Could you check a few things on this drawing? It's one solid part, dimensions in mm from its lowest x, y, z. A direction names the side the tool comes from. Give positions to 0.01 mm unless a question says otherwise; leave off trailing zeros. Order: outer loops, then holes, each group sorted by start corner. A loop starts at its lowest first (then second) coordinate and runs counter-clockwise, first axis right, second up.
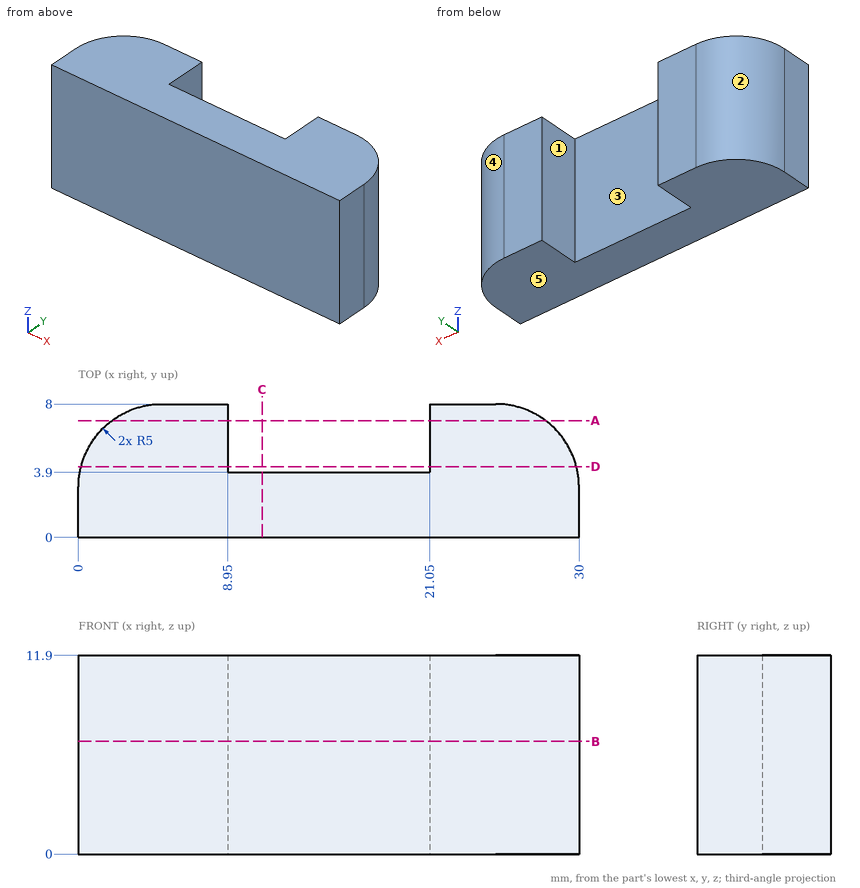
1) Suppose I cut it at C-C (x = 11). Please give me the cut outline in (y, z), and give its area (3 significant figures).
2) Suppose I cut it at A-A (y = 7). Please give me the cut outline in (x, z), and give its area (3 significant figures).
3) Suppose I cut it at D-D (y = 4.25). Please give me the cut outline in (x, z), and give its area (3 significant figures).
4) Which directions (+Z, -Z, +X, -X, +Y, -Y) give clear straight access to the entire face, cutting with the end or side of a thin tool? Please do the marked faces 1 and 2.
5) If I drill on line 1 (Y direction, x = 9.25, z = 5.5); line 2 (X direction, y = 6, z = 1.5); line 3 (X direction, y = 7, z = 11.25), over which ranges is the centre line in solid material (lowest first)?
6) I'm going to push flat-ended pins straight in: pin 1 Ø3.5 at (y, z) = (6, 5) entering from +X; pin 2 Ø4.5 at (y, z) = (5.5, 3) entering from -X; pin 3 Ø3.5 at (x, z) = (16, 6) entering from +Y. Where does each tip first touch, or does it pass through?
7) We'd pull the mould along X, two halves only. Please class the marked faces 3, 4 and 5: +X half, -X half, draft (parallel to the pull), parting line (faces both ways), or undercut.
8) Suppose I cut it at B-B (z = 6.75). Please give me the cut outline in (x, y), and give its area (3 significant figures).
Results:
1. outline: (0, 0) - (3.9, 0) - (3.9, 11.9) - (0, 11.9) - close
1. area: 46.4 mm2
2. outline: (2, 0) - (8.95, 0) - (8.95, 11.9) - (2, 11.9) - close; (21.05, 0) - (28, 0) - (28, 11.9) - (21.05, 11.9) - close
2. area: 165 mm2
3. outline: (0.16, 0) - (8.95, 0) - (8.95, 11.9) - (0.16, 11.9) - close; (21.05, 0) - (29.84, 0) - (29.84, 11.9) - (21.05, 11.9) - close
3. area: 209 mm2
4. face 1: +Z, -Z, +Y
4. face 2: +Z, -Z, -X, +Y
5. line 1: y = 0 to 3.9
5. line 2: x = 1 to 8.95, 21.05 to 29
5. line 3: x = 2 to 8.95, 21.05 to 28
6. pin 1: stops at x = 29.84
6. pin 2: stops at x = 0.01
6. pin 3: stops at y = 3.9
7. face 3: undercut
7. face 4: +X half
7. face 5: draft
8. outline: (0, 0) - (30, 0) - (30, 3) arc R5 ccw to (25, 8) - (21.05, 8) - (21.05, 3.9) - (8.95, 3.9) - (8.95, 8) - (5, 8) arc R5 ccw to (0, 3) - close
8. area: 180 mm2
